Autodesk Inventor part; units mm, degrees
ref_plane "YZ Plane" through (0, 0, 0) normal (1, 0, 0) x (0, 1, 0)
ref_plane "XZ Plane" through (0, 0, 0) normal (0, 1, 0) x (-1, 0, 0)
ref_plane "XY Plane" through (0, 0, 0) normal (0, 0, 1) x (1, 0, 0)
sketch "Sketch4" plane through (0, 0, 0) normal (0, 1, 0) x (-1, 0, 0)
  circle A0 centre (0, 0) radius 39.75
  circle A1 centre (0, 0) radius 41.745
  dimension "d17" = 79.5
  dimension "d18" = 83.49
sketch "Sketch6" plane through (0, 0, 0) normal (0, 1, 0) x (-1, 0, 0)
  circle A0 centre (0, 0) radius 39.7618
extrude "Extrusion1" add sketch "Sketch6" along normal blind 3
extrude "Extrusion2" add sketch "Sketch4" along normal blind 6
sketch "Sketch7" plane through (0, 0, 0) normal (0, -1, 0) x (1, 0, 0)
  circle A0 centre (0, 0) radius 44.86
  circle A1 centre (0, 0) radius 41.6213
extrude "Extrusion3" add sketch "Sketch7" against normal blind 10
sketch "Sketch8" plane through (0, 0, 0) normal (0, -1, 0) x (1, 0, 0)
  circle A0 centre (0, 0) radius 44.86
extrude "Extrusion4" add sketch "Sketch8" along normal blind 1
properties part number "Soft Coating Gripper mold"
Can you work these out from the model? Positions are in its coordinate system, mm. A direction names the side the tool comes from. Coordinates: 2 decimals unless noted, no trailing zeros. Loops run counter-clockwise (first coordinate to the right, second up) from the corner with the lowest first, then second, coordinate; pieces in that order, holes last. Notation, with made-up numbers: M 19,-39.5 L 42,-39.5 A18 cw 42,-8.5 Z; hole C 58.5,-17 d7. An arc over 180 degrees is marked long. Put each result on its own line as item: value. Start each with the question number.
(1) Imagine slicing it at C-C on z = -6.5. List the corners of the cut face in (x, y) for me.
(2) Will these pins go through, and if not, where does the flat tip stop? pin 1 Ø1 at (y, z) = (7.5, 17) entering from +X; pin 2 Ø1 at (x, y) = (0, 1) entering from -Z; pin 3 Ø6 at (y, z) = (7, -16) entering from +X.
(3) Imagine slicing it at A-A on y = 7.75. List the corners of the cut face in (x, z) for me, and give its area (3 significant figures).
(4) Which directions (+Z, -Z, +X, -X, +Y, -Y) give clear straight access to the entire face, cutting with the end or side of a thin tool? Please do faces 1 (the face through (-1, -1, 1)), 2 (the face through (-37, 6, -15)).
(5) Imagine slicing it at D-D on y = 1.5. List the corners of the cut face in (x, z) for me.
(6) I need wall thicknesses on probe 1 along Z at (x, y) = (0, 8); probe 2 along Y at (x, z) = (38, -4); probe 3 along X at (y, z) = (6.75, 32.5). Which ranges of each line are inside material? Lowest first, please.
(7) Imagine slicing it at B-B on x = 0. List the corners of the cut face in (y, z) for me, and give its area (3 significant figures).
(8) We'd pull the mould along Z, two halves only. Please class faces 3 (the face through (1, 3, 1)), 4 (the face through (13, 10, -40)), 5 (the face through (24.116, 4.577, -37.826)): +Z half, -Z half, draft (parallel to the pull), parting line (faces both ways), or undercut.
Worked answers:
1. outline: M -44.39,-1 L 44.39,-1 L 44.39,10 L 41.11,10 L 41.11,6 L 39.21,6 L 39.21,3 L -39.21,3 L -39.21,6 L -41.11,6 L -41.11,10 L -44.39,10 Z
2. pin 1: stops at x = 41.72
2. pin 2: stops at z = -44.86
2. pin 3: stops at x = 42.94
3. outline: C 0,0 d89.72; hole C 0,0 d83.24
3. area: 880 mm2
4. face 1: +Z, -Z, +X, -X, -Y
4. face 2: +Y
5. outline: C 0,0 d89.72
6. probe 1: z = -44.86 to -41.62, 41.62 to 44.86
6. probe 2: y = -1 to 3
6. probe 3: x = -30.92 to -26, 26 to 30.92
7. outline: M -1,-44.86 L 10,-44.86 L 10,-41.62 L 6,-41.62 L 6,-39.75 L 3,-39.75 L 3,39.75 L 6,39.75 L 6,41.62 L 10,41.62 L 10,44.86 L -1,44.86 Z
7. area: 415 mm2
8. face 3: undercut
8. face 4: draft
8. face 5: parting line
